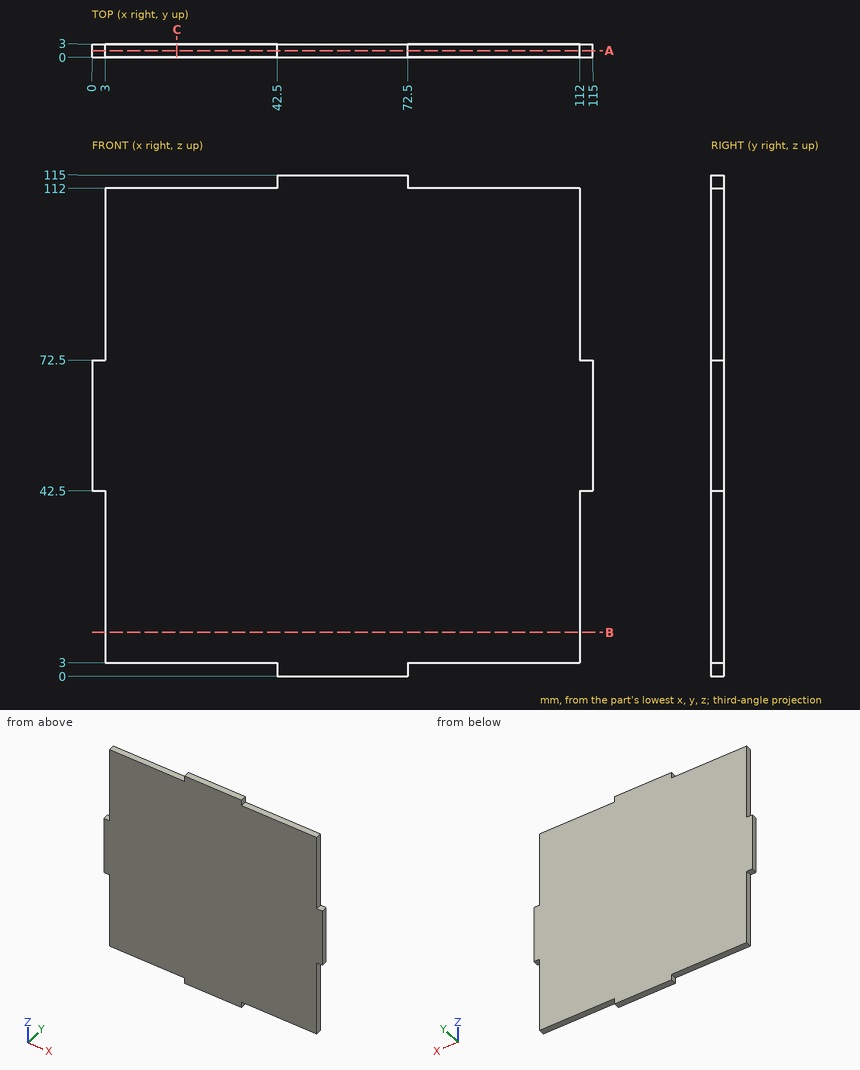
Geometry: see drawing. Coordinates: mm, zero at the bounding-box minimum. Give positions to 0.01 mm unless a question says otherwise; leave off trailing zeros. Order: outer loops, then holes, each group sorted by start corner. A loop starts at its lowest first (then second) coordinate and runs counter-clockwise, first axis right, second up. Notation, with made-up numbers: (-7, 45) - (34, 45) arc R20 ccw to (34, 70) - close; hole circle Ø8 at (69.25, -27). An arc over 180 degrees is marked (long way). Use a Markdown table: item, result.
(1) Pin query (flat end, axial travel): pin 1 (1.5 mm diameter, centred on y = 1, z = 89.5, fed in from -X); pin 2 (0.9 mm diameter, centred on y = 2, z = 84.5, fed in from +X); pin 3 (1.5 mm diameter, centred on x = 94.5, y = 1.5, fed in from -Z). Return the tip coordinate at first contact, or that it passes through.
Computed values:
| item | result |
|---|---|
| pin 1 | stops at x = 3 |
| pin 2 | stops at x = 112 |
| pin 3 | stops at z = 3 |
(2) Section query C-C (x = 19.5). Output: boundary loops of the cut face in (y, z), then the cut area to 3 significant figures.
Computed values:
| item | result |
|---|---|
| outline | (0, 3) - (3, 3) - (3, 112) - (0, 112) - close |
| area | 327 mm2 |
(3) Section query A-A (y = 1.45). Output: boundary loops of the cut face in (x, z), then the cut area to 3 significant figures.
Computed values:
| item | result |
|---|---|
| outline | (0, 42.5) - (3, 42.5) - (3, 3) - (42.5, 3) - (42.5, 0) - (72.5, 0) - (72.5, 3) - (112, 3) - (112, 42.5) - (115, 42.5) - (115, 72.5) - (112, 72.5) - (112, 112) - (72.5, 112) - (72.5, 115) - (42.5, 115) - (42.5, 112) - (3, 112) - (3, 72.5) - (0, 72.5) - close |
| area | 12,200 mm2 |
(4) Section query B-B (z = 10). Output: boundary loops of the cut face in (x, y).
Computed values:
| item | result |
|---|---|
| outline | (3, 0) - (112, 0) - (112, 3) - (3, 3) - close |
(5) Line query: line 1 (Z direction, x = 6, y = 2.85). Output: solid intervals per line, ascending. Write a range as from..to.
Computed values:
| item | result |
|---|---|
| line 1 | z = 3..112 |
